Input: part model. Units: mm. Frame: model coordinates. A direction names the side the tool comes from. Give positions to 0.01 mm unless a question says otherwise; leave off trailing zeros. Loops run counter-clockwise (first coordinate to the right, second up) from the corner with the lowest first, then second, coordinate; pieces in that order, holes last.
from build123d import *

# Parameters (mm, degrees)
BOSS_EXTRUDE2_DEPTH     = 7
CUT_EXTRUDE2_DEPTH      = 30.130224853
CUT_EXTRUDE2_DEPTH_BACK = 30.130224853
SKETCH3_R               = 2
BOSS_EXTRUDE3_DEPTH     = 36
SKETCH5_R               = 2
BOSS_EXTRUDE4_DEPTH     = 7
SKETCH13_W              = 49.8
SKETCH13_H              = 5
BOSS_EXTRUDE6_DEPTH     = 12.25
SKETCH15_W              = 49.8
SKETCH15_H              = 5
BOSS_EXTRUDE7_DEPTH     = 30
BOSS_EXTRUDE8_DEPTH     = 5
FILLET1_DEPTH           = 50
FILLET1_2_DEPTH         = 7
FILLET1_START           = 43
FILLET1_3_DEPTH         = 7
FILLET2_R               = 4
FILLET3_R               = 1
CUT_EXTRUDE3_DEPTH      = 150.305937317
CUT_EXTRUDE3_DEPTH_BACK = 150.305937317
SKETCH16_R              = 1.5
SKETCH16_R_2            = 2.625


with BuildPart() as part:
    # Sketch1 → Boss-Extrude2 (new body)
    with BuildSketch(Plane(origin=(0, 0, 0), x_dir=(1, 0, 0), z_dir=(0, 1, 0))):
        with BuildLine():
            Line((-24.9, 0), (-24.9, 13.4))
            Line((-24.9, 13.4), (24.9, 13.4))
            Line((24.9, 13.4), (24.9, 0))
            ThreePointArc((24.9, 0), (23.392904185, -4.800819919), (19.412411454, -7.878950407))
            Line((19.412411454, -7.878950407), (8.235013612, 1.5))
            ThreePointArc((8.235013612, 1.5), (11.116692467, 6.448255578), (16.5, 8.4))
            Line((16.5, 8.4), (-16.5, 8.4))
            ThreePointArc((-16.5, 8.4), (-11.116692467, 6.448255578), (-8.235013612, 1.5))
            Line((-8.235013612, 1.5), (-19.412411454, -7.878950407))
            ThreePointArc((-19.412411454, -7.878950407), (-23.392904185, -4.800819919), (-24.9, 0))
        make_face()
    extrude(amount=BOSS_EXTRUDE2_DEPTH)

    # Sketch3 → Cut-Extrude2 (cut, two sides: drawn at the far end of the back side and taken through both)
    with BuildSketch(Plane(origin=(0, 7, 0), x_dir=(1, 0, 0), z_dir=(0, 1, 0)).offset(-CUT_EXTRUDE2_DEPTH_BACK)):
        with Locations(Location((-16.5, 0, 0), (0, 0, 270))):
            Circle(SKETCH3_R)
        with Locations(Location((16.5, 0, 0), (0, 0, 270))):
            Circle(SKETCH3_R)
    extrude(amount=CUT_EXTRUDE2_DEPTH + CUT_EXTRUDE2_DEPTH_BACK, mode=Mode.SUBTRACT)

    # Sketch4 → Boss-Extrude3 (add)
    with BuildSketch(Plane(origin=(0, 7, 0), x_dir=(1, 0, 0), z_dir=(0, 1, 0))):
        Polygon((-24.9, 13.4), (-24.9, 0), (-20.9, 0), (-20.9, 8.4), (-16.5, 8.4), (16.5, 8.4), (20.9, 8.4), (20.9, 0), (24.9, 0), (24.9, 13.4), align=None)
    extrude(amount=BOSS_EXTRUDE3_DEPTH)

    # Sketch5 → Boss-Extrude4 (add)
    with BuildSketch(Plane(origin=(0, 43, 0), x_dir=(1, 0, 0), z_dir=(0, 1, 0))):
        with BuildLine():
            Line((-24.9, 13.4), (-24.9, 0))
            ThreePointArc((-24.9, 0), (-23.392904185, -4.800819919), (-19.412411454, -7.878950407))
            Line((-19.412411454, -7.878950407), (-8.235013612, 1.5))
            ThreePointArc((-8.235013612, 1.5), (-11.116692467, 6.448255578), (-16.5, 8.4))
            Line((-16.5, 8.4), (16.5, 8.4))
            ThreePointArc((16.5, 8.4), (11.116692467, 6.448255578), (8.235013612, 1.5))
            Line((8.235013612, 1.5), (19.412411454, -7.878950407))
            ThreePointArc((19.412411454, -7.878950407), (23.392904185, -4.800819919), (24.9, 0))
            Line((24.9, 0), (24.9, 13.4))
            Line((24.9, 13.4), (-24.9, 13.4))
        make_face()
        with Locations(Location((16.5, 0, 0), (0, 0, 270))):
            Circle(SKETCH5_R, mode=Mode.SUBTRACT)
        with Locations(Location((-16.5, 0, 0), (0, 0, 270))):
            Circle(SKETCH5_R, mode=Mode.SUBTRACT)
    extrude(amount=BOSS_EXTRUDE4_DEPTH)

    # Sketch13 → Boss-Extrude6 (add)
    with BuildSketch(Plane(origin=(0, 50, 0), x_dir=(1, 0, 0), z_dir=(0, 1, 0))):
        with Locations((0, 10.9)):
            Rectangle(SKETCH13_W, SKETCH13_H)
    extrude(amount=BOSS_EXTRUDE6_DEPTH)

    # Sketch15 → Boss-Extrude7 (add)
    with BuildSketch(Plane.XZ):
        with Locations((0, -10.9)):
            Rectangle(SKETCH15_W, SKETCH15_H)
    extrude(amount=BOSS_EXTRUDE7_DEPTH)

    # Sketch12 → Boss-Extrude8 (add)
    with BuildSketch(Plane(origin=(0, 0, -13.4), x_dir=(-1, 0, 0), z_dir=(0, 0, -1))):
        Polygon((24.9, -30), (24.9, -41.497235918), (93.105904535, -57.243809722), (79.608841274, -115.706013609), (-67.628165204, -81.713672257), (-54.131101944, -23.25146837), (-24.9, -30), align=None)
    extrude(amount=-BOSS_EXTRUDE8_DEPTH)

    # Fillet1: read off the stored shape, not the designer's step
    # Fillet1 outline → Fillet1 (cut)
    with BuildSketch(Plane(origin=(0, 0, 0), x_dir=(1, 0, 0), z_dir=(0, 1, 0))):
        with BuildLine():
            Line((-19.412411454, -7.878950407), (-17.191978394, -6.015785846))
            ThreePointArc((-17.191978394, -6.015785846), (-20.037614317, -6.942179175), (-22.729609591, -5.63488814))
            ThreePointArc((-22.729609591, -5.63488814), (-21.206707029, -6.957507379), (-19.412411454, -7.878950407))
        make_face()
        with BuildLine():
            ThreePointArc((22.729609591, -5.63488814), (20.037614317, -6.942179175), (17.191978394, -6.015785846))
            Line((17.191978394, -6.015785846), (19.412411454, -7.878950407))
            ThreePointArc((19.412411454, -7.878950407), (21.206707029, -6.957507379), (22.729609591, -5.63488814))
        make_face()
    extrude(amount=FILLET1_DEPTH, mode=Mode.SUBTRACT)

    # Fillet1 2 outline → Fillet1 2 (add)
    with BuildSketch(Plane(origin=(0, 0, 0), x_dir=(1, 0, 0), z_dir=(0, 1, 0))):
        with BuildLine():
            Line((16.5, 8.4), (4.906898603, 8.4))
            ThreePointArc((4.906898603, 8.4), (8.19911817, 6.671847337), (8.646608731, 2.980645161))
            ThreePointArc((8.646608731, 2.980645161), (11.729120592, 6.91366109), (16.5, 8.4))
        make_face()
        with BuildLine():
            ThreePointArc((-16.5, 8.4), (-11.729120592, 6.91366109), (-8.646608731, 2.980645161))
            ThreePointArc((-8.646608731, 2.980645161), (-8.19911817, 6.671847337), (-4.906898603, 8.4))
            Line((-4.906898603, 8.4), (-16.5, 8.4))
        make_face()
    extrude(amount=FILLET1_2_DEPTH)

    # Fillet1 3 outline → Fillet1 3 (add)
    with BuildSketch(Plane(origin=(0, 0, 0), x_dir=(1, 0, 0), z_dir=(0, 1, 0)).offset(FILLET1_START)):
        with BuildLine():
            Line((16.5, 8.4), (4.906898603, 8.4))
            ThreePointArc((4.906898603, 8.4), (8.19911817, 6.671847337), (8.646608731, 2.980645161))
            ThreePointArc((8.646608731, 2.980645161), (11.729120592, 6.91366109), (16.5, 8.4))
        make_face()
        with BuildLine():
            ThreePointArc((-16.5, 8.4), (-11.729120592, 6.91366109), (-8.646608731, 2.980645161))
            ThreePointArc((-8.646608731, 2.980645161), (-8.19911817, 6.671847337), (-4.906898603, 8.4))
            Line((-4.906898603, 8.4), (-16.5, 8.4))
        make_face()
    extrude(amount=FILLET1_3_DEPTH)

    # Fillet2
    fillet2_edges = [part.edges().sort_by_distance(p)[0] for p in [
        (-8.235013612, 3.5, -1.5),
        (8.235013612, 3.5, -1.5),
        (8.235013612, 46.5, -1.5),
        (-8.235013612, 46.5, -1.5),
    ]]
    fillet(fillet2_edges, radius=FILLET2_R)

    # Fillet3
    fillet3_edges = [part.edges().sort_by_distance(p)[0] for p in [
        (-24.9, 25, 0),
        (-20.9, 25, 0),
        (-20.9, 25, -8.4),
        (20.9, 25, -8.4),
        (20.9, 25, 0),
        (24.9, 25, 0),
    ]]
    fillet(fillet3_edges, radius=FILLET3_R)

    # Sketch16 → Cut-Extrude3 (cut, two sides: drawn at the far end of the back side and taken through both)
    with BuildSketch(Plane.XY.offset(-8.4).offset(-CUT_EXTRUDE3_DEPTH_BACK)):
        with Locations((50.684777305, -39.441676722)):
            Circle(SKETCH16_R)
        with Locations((42.889816787, -41.241285157)):
            Circle(SKETCH16_R_2)
        with Locations((44.689425222, -49.036245675)):
            Circle(SKETCH16_R)
        with Locations((35.094856269, -43.040893591)):
            Circle(SKETCH16_R)
        with Locations((41.090208352, -33.446324638)):
            Circle(SKETCH16_R)
        with Locations((-82.911048266, -70.284703313)):
            Circle(SKETCH16_R)
        with Locations((-76.915696183, -60.69013436)):
            Circle(SKETCH16_R)
        with Locations((-67.32112723, -66.685486444)):
            Circle(SKETCH16_R)
        with Locations((-73.316479313, -76.280055397)):
            Circle(SKETCH16_R)
        with Locations((-75.116087748, -68.485094879)):
            Circle(SKETCH16_R_2)
        with Locations(Location((47.838739983, -62.677426582, 0), (0, 0, 180))):
            Circle(SKETCH16_R)
        with Locations(Location((57.433308936, -68.672778665, 0), (0, 0, 180))):
            Circle(SKETCH16_R)
        with Locations(Location((41.843387899, -72.271995535, 0), (0, 0, 180))):
            Circle(SKETCH16_R)
        with Locations(Location((49.638348417, -70.4723871, 0), (0, 0, 180))):
            Circle(SKETCH16_R_2)
        with Locations(Location((51.437956852, -78.267347618, 0), (0, 0, 180))):
            Circle(SKETCH16_R)
        with Locations(Location((-76.162516636, -99.515805257, 0), (0, 0, 180))):
            Circle(SKETCH16_R)
        with Locations(Location((-66.567947683, -105.511157341, 0), (0, 0, 180))):
            Circle(SKETCH16_R)
        with Locations(Location((-60.572595599, -95.916588388, 0), (0, 0, 180))):
            Circle(SKETCH16_R)
        with Locations(Location((-68.367556118, -97.716196822, 0), (0, 0, 180))):
            Circle(SKETCH16_R_2)
        with Locations(Location((-70.167164552, -89.921236304, 0), (0, 0, 180))):
            Circle(SKETCH16_R)
    extrude(amount=CUT_EXTRUDE3_DEPTH + CUT_EXTRUDE3_DEPTH_BACK, mode=Mode.SUBTRACT)


solid = part.part
(1) Ray query, probe 1 along Y at (x, z) = (12.5, -1.5); probe 2 along Z at (x, y) = (-57.5, -91); probe 3 along X at (y, z) = (-20.5, -10.25). Return the intervals inside material, ascending.
Values follow:
probe 1: y = 0 to 7, 43 to 50
probe 2: z = -13.4 to -8.4
probe 3: x = -24.9 to 24.9
(2) Cut plane C-C (x = -55.5). Return the cut outline in (y, z), and give its area (3 significant figures).
Values follow:
outline: (-110.14, -13.4) - (-48.56, -13.4) - (-48.56, -8.4) - (-110.14, -8.4) - close
area: 308 mm2
(3) Pin query (flat end, axial travel): pin 1 Ø4.5 at (x, z) = (16.5, 0) entering from -Y; pin 2 Ø7.5 at (x, z) = (-16.5, -3) entering from +Y; pin 3 Ø1.9 at (y, z) = (23, -5.5) entering from -X. Return the tip coordinate at first contact, or that it passes through.
Values follow:
pin 1: stops at y = 0
pin 2: stops at y = 50
pin 3: stops at x = -24.9
(4) Mould query, pull axis Z, two halves, no side actions, for faces 1 (the flat face through (13.74, 3.45, 3.12)), 2 (the cylindrical face through (18.483, 46.451, -0.26)), 3 (the cylindrical face through (-77.74, -68.37, -10.94)). Classes: +Z half, -Z half, draft (parallel to the pull), parting line (faces both ways), or undercut.
Values follow:
face 1: +Z half
face 2: undercut
face 3: draft
(5) Reachability of faces 4 (the flat face through (-17, 7, -3)), 5 (the cylindrical face through (-8.02, 46.45, -6.91)), 6 (the flat face through (-24.9, 23, -8)), 7 (the cylindrical face through (-19.995, 46.451, 6.945)), 8 (the flat face through (61, -53, -11)) from +Z, -Z, +X, -X, +Y, -Y: full face, straight path, thin tool, end or side. Return the list, or none.
Values follow:
face 4: +Z
face 5: +Y, -Y
face 6: +Z, -Z, -X, +Y
face 7: +Z, +Y, -Y
face 8: +Z, -Z, +X, +Y
(6) Cut plane D-D (y = -85.5). Return the cut outline in (x, z), and give its area (3 significant figures).
Values follow:
outline: (-86.58, -13.4) - (51.23, -13.4) - (51.23, -8.4) - (-86.58, -8.4) - close
area: 689 mm2
(7) Cut plane B-B (z = -11). Count the separate pieces of the cut face and the enclosed holes in it, and give its area (3 significant figures).
Values follow:
separate pieces: 1
enclosed holes: 20
area: 13,700 mm2
(8) Cut plane A-A (y = 13.5). Return the cut outline in (x, z).
Values follow:
outline: (-24.9, -13.4) - (24.9, -13.4) - (24.9, -1) arc R1 ccw to (23.9, 0) - (21.9, 0) arc R1 ccw to (20.9, -1) - (20.9, -7.4) arc R1 cw to (19.9, -8.4) - (-19.9, -8.4) arc R1 cw to (-20.9, -7.4) - (-20.9, -1) arc R1 ccw to (-21.9, 0) - (-23.9, 0) arc R1 ccw to (-24.9, -1) - close
